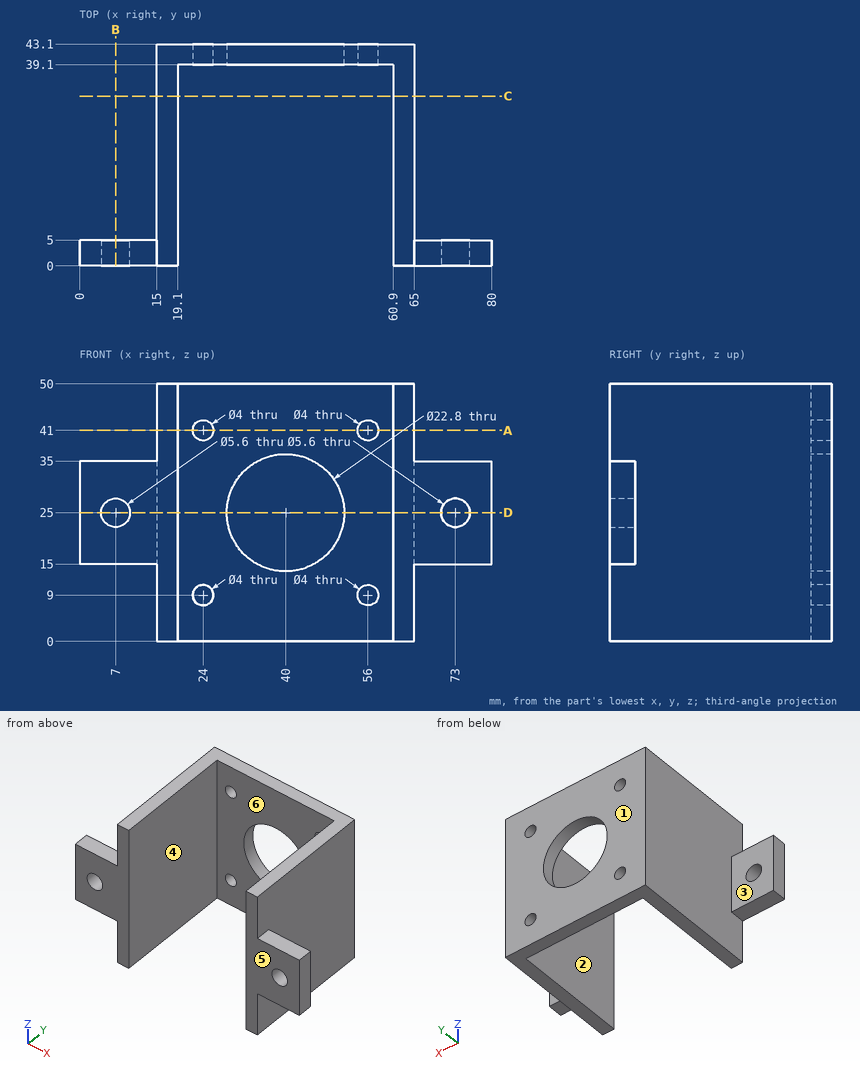
Could you check a few things on this drawing? It's one solid part, dimensions in mm from its lowest x, y, z. A direction names the side the tool comes from. Coordinates: 2 decimals unless noted, no trailing zeros. Loops run counter-clockwise (first coordinate to the right, second up) from the corner with the lowest first, then second, coordinate; pieces in that order, holes last. Notation, with made-up numbers: (77, 44.25) - (111, 44.25) arc R8 ccw to (111, 55.25) - close; hole circle Ø11 at (-8.75, 23). An arc over 180 degrees is marked (long way). Return JSON: item names as keys, results as strings. Group by question number.
Item 1: If we section it at B-B on x = 7: Write out the boundary of the cut face in (y, z).
Item 2: Will these pins go through, and if not, where does the flat tip stop? P1, Ø21, axis at x = 35, z = 31.5, coming from the -Y side; P2, Ø3.5, axis at x = 56, z = 41, coming from the +Y side; P3, Ø13, axis at y = 28, z = 13.5, coming from the +X side; P4, Ø11.5, axis at y = 16.5, z = 20.5, coming from the -X side.
Item 3: On a 3-axis mill with a long thin cutter (end or side, diameter ignored), from which of +Z, -Z, +X, -X, +Y, -Y can I reach the whole of each face in a straight line? I mean the marked faces 1, 2 and 3. Say none if no direction works.
Item 4: We'd pull the mould along X, two halves only. Please class the marked faces 4, 5 and 6: +X half, -X half, draft (parallel to the pull), parting line (faces both ways), or undercut.
Item 5: If we section it at D-D on z = 25: Write out the boundary of the cut face in (x, y).
Item 6: If we section it at A-A on z = 41: Write out the boundary of the cut face in (x, y).
Item 7: I need wall thicknesses on line 1 (X direction, y = 40.2, z = 41); line 2 (Z direction, x = 24, y = 42.2); line 3 (X direction, y = 39, z = 13.5). Which ranges of each line are inside material? Lowest first, please. Write a range as from..to.
Item 8: If we section it at C-C on y = 33: Write out the boundary of the cut face in (x, z).
Calculated:
{
 "1": {"outline": "(0, 15) - (5, 15) - (5, 22.2) - (0, 22.2) - close; (0, 27.8) - (5, 27.8) - (5, 35) - (0, 35) - close"},
 "2": {"P1": "stops at y = 39.1", "P2": "passes through", "P3": "stops at x = 65", "P4": "stops at x = 15"},
 "3": {"face 1": "+Z, -Z, +X, -X, +Y", "face 2": "+Z, -Z, -Y", "face 3": "+Z, -Z, -X, +Y"},
 "4": {"face 4": "undercut", "face 5": "draft", "face 6": "undercut"},
 "5": {"outline": "(0, 0) - (4.2, 0) - (4.2, 5) - (0, 5) - close; (9.8, 0) - (19.1, 0) - (19.1, 39.1) - (28.6, 39.1) - (28.6, 43.1) - (15, 43.1) - (15, 5) - (9.8, 5) - close; (51.4, 39.1) - (60.9, 39.1) - (60.9, 0) - (70.2, 0) - (70.2, 5) - (65, 5) - (65, 43.1) - (51.4, 43.1) - close; (75.8, 0) - (80, 0) - (80, 5) - (75.8, 5) - close"},
 "6": {"outline": "(15, 0) - (19.1, 0) - (19.1, 39.1) - (22, 39.1) - (22, 43.1) - (15, 43.1) - close; (26, 39.1) - (54, 39.1) - (54, 43.1) - (26, 43.1) - close; (58, 39.1) - (60.9, 39.1) - (60.9, 0) - (65, 0) - (65, 43.1) - (58, 43.1) - close"},
 "7": {"line 1": "x = 15..22, 26..54, 58..65", "line 2": "z = 0..7, 11..39, 43..50", "line 3": "x = 15..19.1, 60.9..65"},
 "8": {"outline": "(15, 0) - (19.1, 0) - (19.1, 50) - (15, 50) - close; (60.9, 0) - (65, 0) - (65, 50) - (60.9, 50) - close"}
}
